Work out the finished part from the listing and answer in its coordinate system (mm). Give positions to 0.01 mm unless a question says otherwise; leave off trailing zeros. Write each loop counter-clockwise with the first axis right and the second up, starting at its lowest first coordinate (ties: lowest second). Pieces come first, ordered by that corner, then holes. Notation, with made-up numbers: (70, 51) -> (81, 51) arc R21 ccw to (81, 83) -> close; hole circle Ø7 at (-28.75, -13). An arc over 180 degrees is marked (long way). Use a Markdown table: item, result. Add a question column.
Q1. Section C-C, the plane x = -19 is taken. Give the vertices of the cut face in (y, z).
Q2. Section B-B, the plane z = 29 is taken. State how many separate pieces and enclosed holes the cut face has, plus the area to 3 significant figures.
Q3. Each of these flat-tipped pins is pushed along its axis until it touches: pin 1 Ø8.5 at (x, y) = (0, -21.12) entering from -Z; pin 2 Ø5 at (x, y) = (0, 21.12) entering from +Z. Where does it stop, or does it pass through?
Q4. Consider line 1 (Y direction, x = -20, z = 65.5); line 2 (X direction, y = 17, z = 55); line 3 (Y direction, x = 23, z = 75). Determine where each line is inside the solid, lowest interval first.
Q5. Section A-A, the plane x = 0 is taken. Give the vertices of the cut face in (y, z), plus the area to 3 significant figures.
Q6. Section D-D, the plane x = 42 is taken. Give the vertices of the cut face in (y, z), plus the area to 3 significant figures.
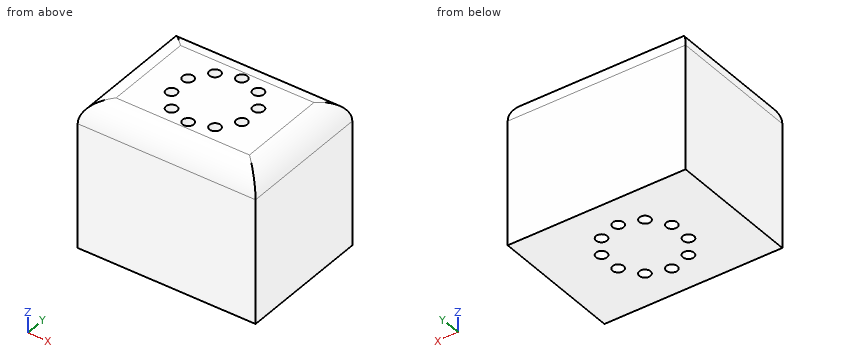
from build123d import *

# Parameters (mm, degrees)
F0_W     = 101.6
F0_H     = 76.2
F1_DEPTH = 83.82
F2_R     = 12.7
F5_D     = 6.35


with BuildPart() as f1:
    # F0 (on Top) → F1 (new body)
    with BuildSketch(Plane.XY):
        Rectangle(F0_W, F0_H)
    extrude(amount=F1_DEPTH)

    # F2
    f2_edges = [f1.edges().sort_by_distance(p)[0] for p in [
        (0, -38.1, 83.82),
        (50.8, 0, 83.82),
        (0, 38.1, 83.82),
        (-50.8, 0, 83.82),
    ]]
    fillet(f2_edges, radius=F2_R)

    # F5 (through all)
    with Locations(Plane.XY.offset(83.82)):
        with Locations((12.416681, -17.090095), (0, -21.124519), (-12.416681, -17.090095), (-20.090612, -6.527835), (-20.090612, 6.527835), (-12.416681, 17.090095), (0, 21.124519), (12.416681, 17.090095), (20.090612, 6.527835), (20.090612, -6.527835)):
            Hole(F5_D / 2)


solid = f1.part
Result set:
| question | item | result |
|---|---|---|
| 1 | outline | (-38.1, 0) -> (-9.51, 0) -> (-9.51, 83.82) -> (-25.4, 83.82) arc R12.7 ccw to (-38.1, 71.12) -> close; (-3.55, 0) -> (3.55, 0) -> (3.55, 83.82) -> (-3.55, 83.82) -> close; (9.51, 0) -> (38.1, 0) -> (38.1, 71.12) arc R12.7 ccw to (25.4, 83.82) -> (9.51, 83.82) -> close |
| 2 | separate pieces | 1 |
| 2 | enclosed holes | 10 |
| 2 | area | 7,430 mm2 |
| 3 | pin 1 | stops at z = 0 |
| 3 | pin 2 | passes through |
| 4 | line 1 | y = -38.1 to -9.7, -3.35 to 3.35, 9.7 to 38.1 |
| 4 | line 2 | x = -50.8 to -15.59, -9.24 to 9.24, 15.59 to 50.8 |
| 4 | line 3 | y = -37.49 to -7.8, -5.26 to 5.26, 7.8 to 37.49 |
| 5 | outline | (-38.1, 0) -> (-24.3, 0) -> (-24.3, 83.82) -> (-25.4, 83.82) arc R12.7 ccw to (-38.1, 71.12) -> close; (-17.95, 0) -> (17.95, 0) -> (17.95, 83.82) -> (-17.95, 83.82) -> close; (24.3, 0) -> (38.1, 0) -> (38.1, 71.12) arc R12.7 ccw to (25.4, 83.82) -> (24.3, 83.82) -> close |
| 5 | area | 5,250 mm2 |
| 6 | outline | (-38.1, 0) -> (38.1, 0) -> (38.1, 71.12) arc R12.7 ccw to (29.3, 83.21) -> (-29.3, 83.21) arc R12.7 ccw to (-38.1, 71.12) -> close |
| 6 | area | 6,280 mm2 |
